Work out the finished part from the listing and answer in its coordinate system (mm). A direction names the side the tool comes from. Give positions to 0.01 mm unless a question says otherwise; leave off trailing zeros. Order: outer loops, then holes, each group sorted by start corner. A loop starts at its lowest first (then second) coordinate and runs counter-clockwise, first axis right, second up. Notation, with made-up numbers: M -1,-34 L 38,-34 A22 ccw 38,-1 Z; hole C 57,50.25 d1. An arc over 180 degrees is marked long. One line per item, written item: value.
from build123d import *

# Parameters (mm, degrees)
F0_R         = 2.125
F1_DEPTH     = 5
F3_DEPTH     = 20
F5_DEPTH     = 15
F6_SIZE      = 10
F7_R         = 2.125
F8_DEPTH     = 5
F9_R         = 2.125
F10_DEPTH    = 5
F11_W        = 40
F11_H        = 20
F11_R        = 2.125
F12_DEPTH    = 24
F13_R        = 4.25
F14_DEPTH    = 25
F15_R        = 3.5
F16_DEPTH    = 25
F17_R        = 4.25
F17_R_2      = 1.6
F18_DEPTH    = 5
F19_T4_DEPTH = 20
F19_S5_R     = 2.125
F19_T6_DEPTH = 12
F19_T7_DEPTH = 36.8584149398
F21_DEPTH    = 12.5
F22_SIZE     = 5
F23_R        = 3.5
F24_DEPTH    = 44.001
F25_R        = 2.125
F26_DEPTH    = 40.001
F28_DEPTH    = 4
F29_R        = 3.5
F30_DEPTH    = 4


# Not quite as in the source:
# - a fillet or chamfer that OpenCascade refuses, or shapes differently, is made with other operations: its cross-section is extruded or revolved along the edge and cut away or added


with BuildPart() as f1:
    # F0 (on Top) → F1 (new body)
    with BuildSketch(Plane.XY):
        Polygon((0, 20), (0, 40), (-20, 40), (-20, 0), (20, 0), (20, 20), align=None)
        with Locations((-7.5, 12.5)):
            Circle(F0_R, mode=Mode.SUBTRACT)
        with Locations((10, 12.5)):
            Circle(F0_R, mode=Mode.SUBTRACT)
        with Locations((-7.5, 30)):
            Circle(F0_R, mode=Mode.SUBTRACT)
    extrude(amount=F1_DEPTH)

    # F2 (on face) → F3 (join)
    with BuildSketch(Plane.XY.offset(5)):
        Polygon((-15, 40), (-20, 40), (-20, 0), (20, 0), (20, 5), (-15, 5), align=None)
    extrude(amount=F3_DEPTH)

    # F4 (on face) → F5 (join)
    with BuildSketch(Plane.XY.offset(25)):
        Polygon((-15, 5), (-15, 25), (-20, 25), (-20, 0), (5, 0), (5, 5), align=None)
    extrude(amount=F5_DEPTH)

    # F6
    f6_edges = [f1.edges().sort_by_distance(p)[0] for p in [
        (0, 20, 2.5),
        (-17.5, 25, 25),
        (5, 2.5, 25),
    ]]
    chamfer(f6_edges, length=F6_SIZE)

    # F7 (on face) → F8 (cut)
    with BuildSketch(Plane.XZ):
        with Locations((-7.5, 32.5)):
            Circle(F7_R)
        with Locations((10, 12.5)):
            Circle(F7_R)
    extrude(amount=-F8_DEPTH, mode=Mode.SUBTRACT)

    # F9 (on face) → F10 (cut)
    with BuildSketch(Plane(origin=(-20, 0, 0), x_dir=(0, -1, 0), z_dir=(-1, 0, 0))):
        with Locations((-12.5, 32.5)):
            Circle(F9_R)
        with Locations((-30, 12.5)):
            Circle(F9_R)
    extrude(amount=-F10_DEPTH, mode=Mode.SUBTRACT)

    # F11 (on face) → F12 (join)
    with BuildSketch(Plane(origin=(0, 0, 0), x_dir=(1, 0, 0), z_dir=(0, 0, -1))):
        with Locations((0, -10)):
            Rectangle(F11_W, F11_H)
        with Locations((-7.5, -12.5)):
            Circle(F11_R, mode=Mode.SUBTRACT)
        with Locations((10, -12.5)):
            Circle(F11_R, mode=Mode.SUBTRACT)
    extrude(amount=F12_DEPTH)

    # F13 (on face) → F14 (cut)
    with BuildSketch(Plane(origin=(0, 20, 0), x_dir=(-1, 0, 0), z_dir=(0, 1, 0))):
        with Locations((7.5, -11.5)):
            Circle(F13_R)
        Polygon((-5, -24), (-5, -11.5), (-5, 0), (-20, 0), (-20, -24), align=None)
    extrude(amount=-F14_DEPTH, mode=Mode.SUBTRACT)

    # F15 (on face) → F16 (cut)
    with BuildSketch(Plane(origin=(0, 0, 0), x_dir=(1, 0, 0), z_dir=(0, 0, -1))):
        with Locations((-7.5, -12.5)):
            Circle(F15_R)
    extrude(amount=F16_DEPTH, mode=Mode.SUBTRACT)

    # F17 (on face) → F18 (join)
    with BuildSketch(Plane.XZ):
        with Locations((-7.5, -11.5)):
            Circle(F17_R)
        with Locations((-7.5, -11.5)):
            Circle(F17_R_2, mode=Mode.SUBTRACT)
    extrude(amount=-F18_DEPTH)

    # F19: chamfer of 5 on 2 edges, made by hand


with BuildPart() as f19_tool2:
    # F19_s3 → F19_t4 (new body)
    with BuildSketch(Plane.XZ.offset(-20)):
        Polygon((5, -5), (10, 0), (5, 0), align=None)
    extrude(amount=F19_T4_DEPTH)

    # F19_s5 → F19_t6 (cut, symmetric)
    with BuildSketch(Plane.XY.offset(-2.5)):
        with Locations((10, 12.5)):
            Circle(F19_S5_R)
    extrude(amount=F19_T6_DEPTH, both=True, mode=Mode.SUBTRACT)


with BuildPart() as f1_1:
    add(f1.part)

    # F19_t1: union F19_tool2
    add(f19_tool2.part)

    # F19_s8 → F19_t7 (cut)
    with BuildSketch(Plane.XY.offset(-36.8584149398)):
        Polygon((-20, 15), (-15, 20), (-20, 20), align=None)
    extrude(amount=F19_T7_DEPTH, mode=Mode.SUBTRACT)

    # F20 (on face) → F21 (join)
    with BuildSketch(Plane.XZ):
        Polygon((-12.25, -24), (-20, -24), (-20, -44), (5, -44), (5, -24), (-2.75, -24), (-2.75, -39), (-12.25, -39), align=None)
    extrude(amount=-F21_DEPTH)

    # F22
    f22_edges = [f1_1.edges().sort_by_distance(p)[0] for p in [
        (-20, 6.25, -44),
        (5, 6.25, -44),
        (5, 20, -14.5),
    ]]
    chamfer(f22_edges, length=F22_SIZE)

    # F23 (on face) → F24 (cut, through all)
    with BuildSketch(Plane(origin=(0, 0, 0), x_dir=(1, 0, 0), z_dir=(0, 0, -1))):
        with Locations((10, -12.5)):
            Circle(F23_R)
    extrude(amount=F24_DEPTH, mode=Mode.SUBTRACT)

    # F25 (on face) → F26 (cut, through all)
    with BuildSketch(Plane(origin=(-20, 0, 0), x_dir=(0, -1, 0), z_dir=(-1, 0, 0))):
        with Locations((-6.25, -31.5)):
            Circle(F25_R)
    extrude(amount=-F26_DEPTH, mode=Mode.SUBTRACT)

    # F27 (on face) → F28 (cut)
    with BuildSketch(Plane(origin=(-20, 0, 0), x_dir=(0, -1, 0), z_dir=(-1, 0, 0))):
        Polygon((-3.325, -33.1887495374), (-3.325, -29.8112504626), (-6.25, -28.1225009252), (-9.175, -29.8112504626), (-9.175, -33.1887495374), (-6.25, -34.8774990748), align=None)
    extrude(amount=-F28_DEPTH, mode=Mode.SUBTRACT)

    # F29 (on face) → F30 (cut)
    with BuildSketch(Plane.YZ.offset(5)):
        with Locations((6.25, -31.5)):
            Circle(F29_R)
    extrude(amount=-F30_DEPTH, mode=Mode.SUBTRACT)


solid = f1_1.part
(1) Section B-B, the plane z = 12.5 is taken. Give the vertices of the cut face in (x, y) (3 decimals), then the cut area to 4 significant figures.
Findings:
outline: M -20,0 L 7.875,0 L 7.875,5 L -15,5 L -15,27.875 L -20,27.875 Z; M -20,32.125 L -15,32.125 L -15,40 L -20,40 Z; M 12.125,0 L 20,0 L 20,5 L 12.125,5 Z
area: 332.5 mm^2
(2) Which of the six approach directions +Z, -Z, +X, -X, +Y, -Y give full straight-line access (tool end or side, diameter ignored) to faces 4 (the flat face through (-12.25, 4.8, -33.3)), 5 (the cylindrical face through (-4.267, 13.841, -4.481)), 6 (the flat face through (-18.028, 7.733, -34.021)), 7 (the cylindrical face through (-6.519, 14.385, 2.535)), 8 (the flat face through (-4.9, 9.9, -24))?
Findings:
face 4: +Y, -Y
face 5: none
face 6: -X
face 7: +Z
face 8: +Y
(3) Section A-A, the plane z = -31.5 is taken. Give the vertices of the cut face in (x, y) (3 decimals), then the cut area to 3 significant figures.
Findings:
outline: M -20,0 L -12.25,0 L -12.25,4.125 L -16,4.125 L -16,3.325 L -20,3.325 Z; M -20,9.175 L -16,9.175 L -16,8.375 L -12.25,8.375 L -12.25,12.5 L -20,12.5 Z; M -2.75,0 L 5,0 L 5,2.75 L 1,2.75 L 1,4.125 L -2.75,4.125 Z; M -2.75,8.375 L 1,8.375 L 1,9.75 L 5,9.75 L 5,12.5 L -2.75,12.5 Z
area: 110 mm^2
(4) Find the intervals of material crossed by probe 1 along Z at (x, y) = (-18.2, 30) (3 decimals); probe 2 along X at (y, z) = (12, 2); probe 3 along Z at (x, y) = (-0.5, 17.5), in increasing order. Write a range as from..to.
Findings:
probe 1: z = 0..10.375, 14.625..30
probe 2: x = -20..-9.57, -5.43..7.93, 12.07..20
probe 3: z = -24..5
(5) Determine the mould class of faces 1 (the flat face through (-7, 6, -39)), 2 (the flat face through (-17, 40, 7)), 3 (the flat face through (-18, 38, 25)) for opening direction Z: pulls with the +Z half, pulls with the -Z half, needs draft (parallel to the pull), parting line crosses it, or undercut.
Findings:
face 1: undercut
face 2: needs draft
face 3: pulls with the +Z half
(6) Given P1, Ø5, axis at x = -13.5, z = 21, coming from the -Y side; P2, Ø12.5, axis at x = -8.5, y = 24, coming from the -Z side; P3, Ø5.5, axis at x = 18, y = 3.5, coming from the +Z side; P4, Ø4, axis at x = 5, y = 10.5, coming from the +Z side, each flat-ended and moving along its own axis, determine where each tip first touches the part or whether it passes through.
Findings:
P1: stops at y = 0
P2: stops at z = -24
P3: stops at z = 25
P4: stops at z = 5
(7) Section C-C, the plane z = -6 is taken. Give the vertices of the cut face in (x, y).
Findings:
outline: M -20,0 L 5,0 L 5,15 L 4,16 L 4,20 L -15,20 L -20,15 Z; hole C -7.5,12.5 d7
(8) Section D-D, the plane x = 9 is taken. Give the vertices of the cut face in (y, z) (3 decimals).
Findings:
outline: M 0,-1 L 9.146,-1 L 9.146,0 L 10.625,0 L 10.625,5 L 5,5 L 5,10.625 L 0,10.625 Z; M 0,14.375 L 5,14.375 L 5,31 L 0,31 Z; M 14.375,0 L 15.854,0 L 15.854,-1 L 20,-1 L 20,0 L 21,0 L 21,5 L 14.375,5 Z
